```python
from build123d import *

# Parameters (mm, degrees)
PCB_DIMENSIONS_W    = 47.716732244
PCB_DIMENSIONS_H    = 81.636732244
BOSS_EXTRUDE3_DEPTH = 1.5
SKETCH5_W           = 43.474091557
SKETCH5_H           = 77.394091557
SKETCH5_W_2         = 39.23145087
SKETCH5_H_2         = 73.15145087
BOSS_EXTRUDE4_DEPTH = 1.8
FILLET1_R           = 1
SKETCH6_W           = 12
SKETCH6_H           = 29.966906412
SKETCH6_H_2         = 34.033093588
BOSS_EXTRUDE5_DEPTH = 10
SKETCH7_W           = 48
SKETCH7_H           = 6
CUT_EXTRUDE1_DEPTH  = 24
FILLET2_R           = 6
FILLET3_R           = 1
SCALE1_SCALE        = 0.99
CUT_EXTRUDE2_DEPTH  = 10
SKETCH9_R           = 2.4
CUT_EXTRUDE3_DEPTH  = 10


with BuildPart() as part:
    # PCB Dimensions → Boss-Extrude3 (new body)
    with BuildSketch(Plane(origin=(0, 0, 0), x_dir=(1, 0, 0), z_dir=(0, 1, 0))):
        with Locations((20.322832216, -37.282832216)):
            Rectangle(PCB_DIMENSIONS_W, PCB_DIMENSIONS_H)
    extrude(amount=BOSS_EXTRUDE3_DEPTH)

    # Sketch5 → Boss-Extrude4 (add)
    with BuildSketch(Plane(origin=(0, 1.5, 0), x_dir=(1, 0, 0), z_dir=(0, 1, 0))):
        with Locations((20.322832217, -37.282832217)):
            Rectangle(SKETCH5_W, SKETCH5_H)
        with Locations((20.322832216, -37.282832216)):
            Rectangle(SKETCH5_W_2, SKETCH5_H_2, mode=Mode.SUBTRACT)
    extrude(amount=BOSS_EXTRUDE4_DEPTH)

    # Fillet1
    fillet1_edges = [part.edges().sort_by_distance(p)[0] for p in [
        (-1.414213562, 2.4, -1.414213562),
        (-1.414213562, 2.4, 75.979877995),
        (42.059877995, 2.4, 75.979877995),
        (42.059877995, 2.4, -1.414213562),
        (0.707106781, 2.4, 0.707106781),
        (0.707106781, 2.4, 73.858557651),
        (39.938557651, 2.4, 73.858557651),
        (39.938557651, 2.4, 0.707106781),
    ]]
    fillet(fillet1_edges, radius=FILLET1_R)

    # Sketch6 → Boss-Extrude5 (add)
    with BuildSketch(Plane.XZ):
        with Locations((14.322832216, 52.266285422)):
            Rectangle(SKETCH6_W, SKETCH6_H)
        with Locations((26.322832216, 52.266285422)):
            Rectangle(SKETCH6_W, SKETCH6_H)
        with Locations((14.322832216, 20.266285422)):
            Rectangle(SKETCH6_W, SKETCH6_H_2)
        with Locations((26.322832216, 20.266285422)):
            Rectangle(SKETCH6_W, SKETCH6_H_2)
    extrude(amount=BOSS_EXTRUDE5_DEPTH)

    # Sketch7 → Cut-Extrude1 (cut)
    with BuildSketch(Plane(origin=(32.322832216, 0, 0), x_dir=(0, 0, -1), z_dir=(1, 0, 0))):
        with Locations((-35.249738628, -3)):
            Rectangle(SKETCH7_W, SKETCH7_H)
    extrude(amount=-CUT_EXTRUDE1_DEPTH, mode=Mode.SUBTRACT)

    # Fillet2
    fillet2_edges = [part.edges().sort_by_distance(p)[0] for p in [
        (20.322832216, -10, 67.249738628),
        (20.322832216, -10, 3.249738628),
    ]]
    fillet(fillet2_edges, radius=FILLET2_R)

    # Fillet3
    fillet3_edges = [part.edges().sort_by_distance(p)[0] for p in [
        (20.322832216, -6, 59.249738628),
        (20.322832216, -6, 11.249738628),
    ]]
    fillet(fillet3_edges, radius=FILLET3_R)


with BuildPart() as part_1:
    # Scale1: scaled about (20.322832216, -3.130115188, 36.173441116)
    add(part.part.scale(SCALE1_SCALE).moved(Location((0.203228322, -0.031301152, 0.361734411))))

    # Sketch8 → Cut-Extrude2 (cut)
    with BuildSketch(Plane.XZ.offset(0.031301152)):
        Polygon((20.322832216, 77.681920766), (12.322832216, 77.681920766), (12.322832216, 66.938975653), (28.322832216, 66.938975653), (28.322832216, 77.681920766), align=None)
    extrude(amount=-CUT_EXTRUDE2_DEPTH, mode=Mode.SUBTRACT)

    # Sketch9 → Cut-Extrude3 (cut)
    with BuildSketch(Plane.XZ.offset(0.031301152)):
        with Locations((1.373049755, 60.612830152)):
            Circle(SKETCH9_R)
    extrude(amount=-CUT_EXTRUDE3_DEPTH, mode=Mode.SUBTRACT)


solid = part_1.part
```
Work out the finished part from the listing and answer in its coordinate system (mm). A direction names the side the tool comes from. Give positions to 0.01 mm unless a question says otherwise; leave off trailing zeros. Order: outer loops, then holes, each group sorted by start corner. A loop starts at its lowest first (then second) coordinate and runs counter-clockwise, first axis right, second up. Notation, with made-up numbers: (18, -8) - (27, -8) arc R33 ccw to (27, 21) - close; hole circle Ø4 at (-39.75, 13.25). An arc over 180 degrees is marked (long way). One line per item, written item: value. Start each with the question number.
1. Which of the six approach directions +Z, -Z, +X, -X, +Y, -Y give full straight-line access (tool end or side, diameter ignored) to faces 1 (the face through (20, -3, 59.019)), 2 (the face through (-1.197, 2, 38)), 3 (the face through (7, 2, 73.482))?
2. Consider line 1 (Z direction, x = 31, y = 2); line 2 (Z direction, x = 9, y = -1.75); line 3 (Y direction, x = 28.5, z = 16.5). Determine where each line is inside the solid, lowest interval first.
3. Section C-C, the plane x = 11 is taken. Write down the section's boundary in (y, z), then the cut area to 3 significant figures.
4. Section B-B, the plane z = 20 is taken. Write down the section's boundary in (x, y).
5. Section D-D, the plane x = 6 is taken. Write down the section's boundary in (y, z).
6. Section A-A, the plane y = -3 is taken. Write down the section's boundary in (x, z).
7. For a pull along Z with two mould halves and no side action, classify faces 4 (the face through (6, 2, 75.582)), 5 (the face through (20, -3, 11.499)), 6 (the face through (20.489, -8.145, 5.273)), 7 (the face through (20, -9.931, 36)) as released by +Z, released by -Z, zero draft, split by the parting line, or undercut.
8. Each of these flat-tipped pins is pushed along its axis until it touches: pin 1 Ø4 at (x, y) = (25, -1.5) entering from +Z; pin 2 Ø5 at (y, z) = (-5, 34) entering from +X; pin 3 Ø2.5 at (x, y) = (26, -3.5) entering from -Z. Where does it stop, or does it pass through?
Filled sheet:
1. face 1: +X, -X
1. face 2: +Z, -Z, -X, +Y
1. face 3: +Y
2. line 1: -1.04 to 1.06, 73.48 to 75.58
2. line 2: 3.58 to 11.5, 59.02 to 66.94
2. line 3: -9.93 to -5.97, -0.03 to 1.45
3. outline: (-9.93, 9.52) arc R5.94 ccw to (-3.99, 3.58) - (-0.03, 3.58) - (-0.03, -3.14) - (1.45, -3.14) - (1.45, -1.04) - (3.24, -1.04) - (3.24, 1.06) - (1.45, 1.06) - (1.45, 73.48) - (3.24, 73.48) - (3.24, 75.58) - (1.45, 75.58) - (1.45, 77.68) - (-0.03, 77.68) - (-0.03, 66.94) - (-3.99, 66.94) arc R5.94 ccw to (-9.93, 61) - close; hole (-5.97, 12.49) arc R0.99 ccw to (-4.98, 11.5) - (-0.03, 11.5) - (-0.03, 59.02) - (-4.98, 59.02) arc R0.99 ccw to (-5.97, 58.03) - close
3. area: 458 mm²
4. outline: (-3.3, -0.03) - (43.94, -0.03) - (43.94, 1.45) - (41.84, 1.45) - (41.84, 3.24) - (39.74, 3.24) - (39.74, 1.45) - (0.9, 1.45) - (0.9, 3.24) - (-1.2, 3.24) - (-1.2, 1.45) - (-3.3, 1.45) - close; (8.44, -9.93) - (32.2, -9.93) - (32.2, -5.97) - (8.44, -5.97) - close
5. outline: (-0.03, -3.14) - (1.45, -3.14) - (1.45, -1.04) - (3.24, -1.04) - (3.24, 1.06) - (1.45, 1.06) - (1.45, 73.48) - (3.24, 73.48) - (3.24, 75.58) - (1.45, 75.58) - (1.45, 77.68) - (-0.03, 77.68) - close
6. outline: (8.44, 3.58) - (32.2, 3.58) - (32.2, 11.5) - (8.44, 11.5) - close; (8.44, 59.02) - (32.2, 59.02) - (32.2, 66.94) - (8.44, 66.94) - close
7. face 4: released by +Z
7. face 5: undercut
7. face 6: released by -Z
7. face 7: zero draft
8. pin 1: z = 66.94
8. pin 2: x = 32.2
8. pin 3: z = 3.58
